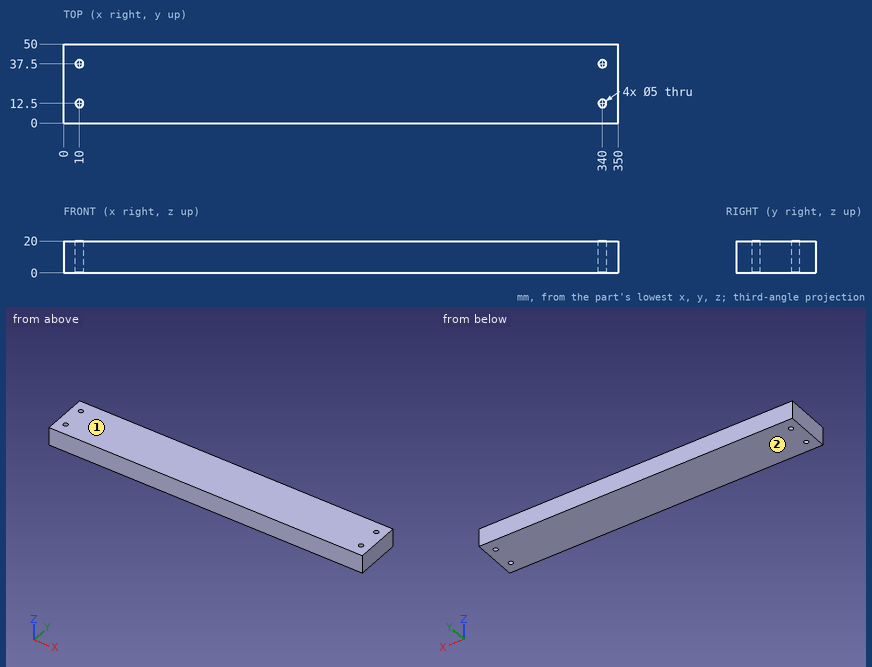
Could you check a few things on this drawing? It's one solid part, dimensions in mm from its lowest x, y, z. Give positions to 0.01 mm unless a question says otherwise; leave off trailing zeros. Answer as CSV lines item,"result". Start each with the question number.
(1) I'm going to push a flat-ended pin straight in: pin 1 Ø3 at (x, y) = (340, 37.5) entering from +Z. Where does the tip first touch, or does it pass through?
(2) Please list where these lines run through material, in increasing order: line 1 (Y direction, x = 340, z = 13); line 2 (X direction, y = 14.5, z = 16.75); line 3 (X direction, y = 11, z = 1.5).
(3) If we mould it in two halves opening along Z, with no side actions, what happens to the marked faces 1 and 2? For each: +Z half, -Z half, draft (parallel to the pull), parting line (faces both ways), or undercut.
Answer list:
1,pin 1,"through"
2,line 1,"0 to 10, 15 to 35, 40 to 50"
2,line 2,"0 to 8.5, 11.5 to 338.5, 341.5 to 350"
2,line 3,"0 to 8, 12 to 338, 342 to 350"
3,face 1,"+Z half"
3,face 2,"-Z half"
